For this review, use the dimensioned drawing (mm, ordinates from the lowest corner) and the shaded views. Coordinates: 2 decimals unless noted, no trailing zeros. Loops run counter-clockwise (first coordinate to the right, second up) from the corner with the lowest first, then second, coordinate; pieces in that order, holes last. Notation, with made-up numbers: (82.25, 43) - (111.25, 43) arc R21 cw to (111.25, 72) - close; hole circle Ø11 at (46, 32). An arc over 180 degrees is marked (long way). Answer in a Markdown table with one row per item. Add a question column.
(1) We need section C-C on y = 8. Write out the cut boundary in (x, z).
(2) For P1, Ø4, axis at x = 103, y = 8, coming from the +Z side, flat-tipped, find the tip position at first contact; note if it passes through.
(3) We need section A-A on x = 15. Write out the cut boundary in (y, z), plus the area to 3 significant figures.
(4) We need section D-D on z = 3.5. Give the number of separate pieces and of enclosed holes in the cut face, plus the area to 3 significant figures.
(5) For line 1 along Y through (x, z) = (135, 2); line 2 along Y through (x, z) = (75, 2.5); line 3 along X through (y, z) = (60, 6.5), list the stretches that pass through material, from the lowest coordinate up.
(6) We need section B-B on x = 75. Write out the cut boundary in (y, z), plus the area to 3 significant figures.
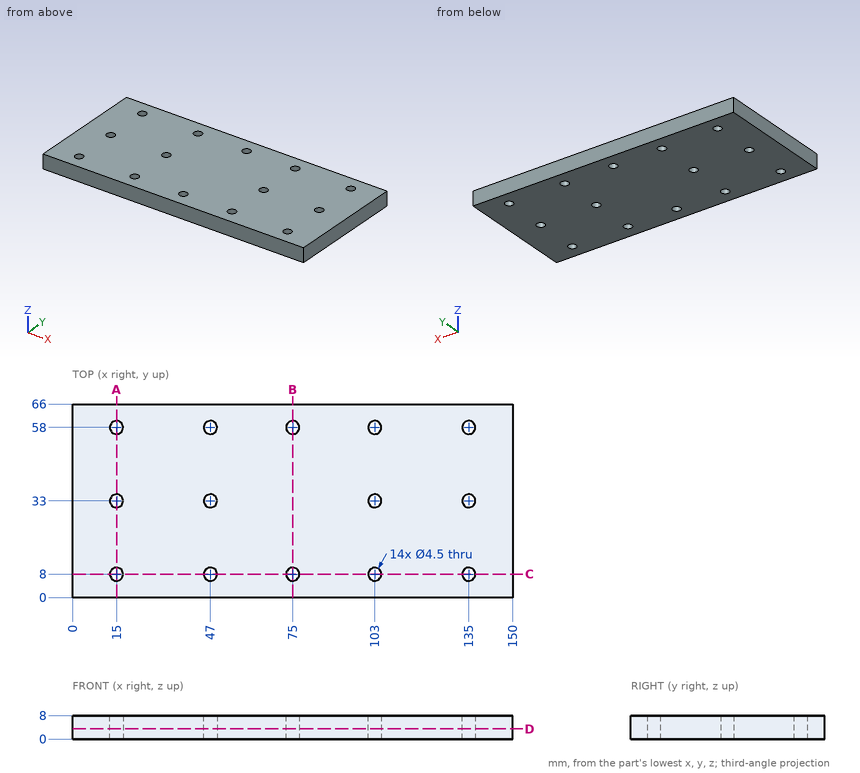
Outcome:
| question | item | result |
|---|---|---|
| 1 | outline | (0, 0) - (12.75, 0) - (12.75, 8) - (0, 8) - close; (17.25, 0) - (44.75, 0) - (44.75, 8) - (17.25, 8) - close; (49.25, 0) - (72.75, 0) - (72.75, 8) - (49.25, 8) - close; (77.25, 0) - (100.75, 0) - (100.75, 8) - (77.25, 8) - close; (105.25, 0) - (132.75, 0) - (132.75, 8) - (105.25, 8) - close; (137.25, 0) - (150, 0) - (150, 8) - (137.25, 8) - close |
| 2 | P1 | through |
| 3 | outline | (0, 0) - (5.75, 0) - (5.75, 8) - (0, 8) - close; (10.25, 0) - (30.75, 0) - (30.75, 8) - (10.25, 8) - close; (35.25, 0) - (55.75, 0) - (55.75, 8) - (35.25, 8) - close; (60.25, 0) - (66, 0) - (66, 8) - (60.25, 8) - close |
| 3 | area | 420 mm² |
| 4 | separate pieces | 1 |
| 4 | enclosed holes | 14 |
| 4 | area | 9,680 mm² |
| 5 | line 1 | 0 to 5.75, 10.25 to 30.75, 35.25 to 55.75, 60.25 to 66 |
| 5 | line 2 | 0 to 5.75, 10.25 to 55.75, 60.25 to 66 |
| 5 | line 3 | 0 to 13.97, 16.03 to 45.97, 48.03 to 73.97, 76.03 to 101.97, 104.03 to 133.97, 136.03 to 150 |
| 6 | outline | (0, 0) - (5.75, 0) - (5.75, 8) - (0, 8) - close; (10.25, 0) - (55.75, 0) - (55.75, 8) - (10.25, 8) - close; (60.25, 0) - (66, 0) - (66, 8) - (60.25, 8) - close |
| 6 | area | 456 mm² |
